Input: part model. Units: mm. Frame: model coordinates. Face numbers are marked on the shaded views. A direction names the side the tool comes from. Give positions to 0.01 mm unless a question says otherwise; leave off trailing zeros. Loops run counter-clockwise (first coordinate to the right, second up) from the corner with the lowest first, then second, coordinate; pieces in that order, holes last. Notation, with made-up numbers: (-34, 20.25) - (6, 20.25) arc R31 cw to (6, 56.25) - close; hole circle Ø3 at (-12, 72.5). An arc over 180 degrees is marked (long way). Answer as a JSON object with one key per item and string values. Group by question number.
(1) Access query for the marked faces 4, 5 and 6. Directions: +Z, -Z, +X, -X, +Y, -Y. A direction counts if a zero-diameter tool reaches every point of the face in a straight line with its end or side. Return the directions, or none.
(2) Section query A-A (y = -28). Return loops of the section in (x, z).
(3) Material intervals for L1, parallel to Z at x = 40.5, y = -23.5; L2, parallel to X at y = -10, z = 9.25; L3, parallel to Z at x = 72, y = 13.5, sorted ascending.
(4) Section query D-D (x = 23.5). Return loops of the section in (y, z).
(5) Section query C-C (y = 44). Return loops of the section in (x, z), plus the area to 3 significant figures.
(6) Pin query (flat end, axial travel): P1, Ø5, axis at x = 5.5, z = 18.5, coming from the -Y side; P2, Ø1.5, axis at y = 22.5, z = 22.5, coming from the -X side; P3, Ø8.5, axis at x = 60.85, y = 12.86, coming from the +Z side. Return the tip coordinate at first contact, or that it passes through.
(7) Section query B-B (z = 16). Return loops of the section in (x, y), plus the area to 3 significant figures.
(8) Mould query, pull axis Z, two halves, no side actions, for the marked faces 1, 2 and 3. Classes: +Z half, -Z half, draft (parallel to the pull), parting line (faces both ways), or undercut.
```python
from build123d import *

# Parameters (mm, degrees)
F1_DEPTH     = 25
F4_DEPTH     = 25
F6_DEPTH     = 20
F7_W         = 51.9104144033
F7_H         = 33.7755738664
F7_W_2       = 52.9833799657
F8_DEPTH     = 25
F9_W         = 5
F9_H         = 24.4488522671
F10_DEPTH    = 20
F11_W        = 120.8302378654
F11_H        = 15
F12_DEPTH    = 30
F14_DEPTH    = 6
F15_R        = 7.2754238601
F15_R_2      = 3.5
F15_R_3      = 6.751082942
F16_DEPTH    = 2
F17_W        = 5
F17_H        = 5
F18_DEPTH    = 58
F19_DEPTH    = 2
F20_T1_DEPTH = 5
F20_T3_DEPTH = 5
F20_T5_DEPTH = 50
F20_T7_DEPTH = 30
F20_T9_DEPTH = 30


# Not quite as in the source:
# - a fillet or chamfer that OpenCascade refuses, or shapes differently, is made with other operations: its cross-section is extruded or revolved along the edge and cut away or added
# - a feature names something its author has since deleted; it is built from what else it names


with BuildPart() as f1:
    # F0 (on Top) → F1 (new body)
    with BuildSketch(Plane.XY):
        Polygon((-25, 55.486739397), (-90.4999962505, 55.486739397), (-90.4999962505, -36.513260603), (90.5000037495, -36.513260603), (90.5000037495, 55.486739397), (25, 55.486739397), align=None)
    extrude(amount=F1_DEPTH)

    # F3 (on face) → F4 (cut)
    with BuildSketch(Plane.XY.offset(25)):
        Polygon((10, -17.952421695), (0, -17.952421695), (-10, -17.952421695), (-10, -30.3189372783), (0, -30.3189372783), (10, -30.3189372783), align=None)
        Polygon((10, -36.513260603), (10, -30.3189372783), (0, -30.3189372783), (-10, -30.3189372783), (-10, -36.513260603), align=None)
    extrude(amount=-F4_DEPTH, mode=Mode.SUBTRACT)

    # F5 (on face) → F6 (cut)
    with BuildSketch(Plane.XY.offset(25)):
        Polygon((83.3136215806, -2.7376867365), (83.3136215806, 55.486739397), (-90.4999962505, 55.486739397), (-90.4999962505, -36.513260603), (-37.5166162848, -36.513260603), (-37.5166162848, -2.7376867365), align=None)
    extrude(amount=-F6_DEPTH, mode=Mode.SUBTRACT)

    # F7 (on face) → F8 (cut)
    with BuildSketch(Plane.XY.offset(5)):
        with Locations((-64.5447890489, 38.5989524638)):
            Rectangle(F7_W, F7_H)
        with Locations((-64.0083062677, -19.6254736697)):
            Rectangle(F7_W_2, F7_H)
    extrude(amount=-F8_DEPTH, mode=Mode.SUBTRACT)

    # F9 (on face) → F10 (join)
    with BuildSketch(Plane.XY.offset(5)):
        with Locations((-87.9999962505, 9.486739397)):
            Rectangle(F9_W, F9_H)
    extrude(amount=F10_DEPTH)

    # F11 (on face) → F12 (cut)
    with BuildSketch(Plane(origin=(0, -2.7376867365, 0), x_dir=(-1, 0, 0), z_dir=(0, 1, 0))):
        with Locations((-22.8985026479, 12.5)):
            Rectangle(F11_W, F11_H)
    extrude(amount=-F12_DEPTH, mode=Mode.SUBTRACT)

    # F13 (on face) → F14 (cut)
    with BuildSketch(Plane.XY.offset(5)):
        with BuildLine():
            ThreePointArc((64.3544293493, 12.8630390391), (60.8544293493, 16.3630390391), (57.3544293493, 12.8630390391))
            Line((57.3544293493, 12.8630390391), (60.8544293493, 12.8630390391))
            Line((60.8544293493, 12.8630390391), (64.3544293493, 12.8630390391))
        make_face()
        with BuildLine():
            Line((60.8544293493, 12.8630390391), (57.3544293493, 12.8630390391))
            ThreePointArc((57.3544293493, 12.8630390391), (60.8544293493, 9.3630390391), (64.3544293493, 12.8630390391))
            Line((64.3544293493, 12.8630390391), (60.8544293493, 12.8630390391))
        make_face()
        with BuildLine():
            ThreePointArc((-23.8955706507, 12.8630390391), (-27.3955706507, 16.3630390391), (-30.8955706507, 12.8630390391))
            Line((-30.8955706507, 12.8630390391), (-27.3955706507, 12.8630390391))
            Line((-27.3955706507, 12.8630390391), (-23.8955706507, 12.8630390391))
        make_face()
        with BuildLine():
            Line((-27.3955706507, 12.8630390391), (-30.8955706507, 12.8630390391))
            ThreePointArc((-30.8955706507, 12.8630390391), (-27.3955706507, 9.3630390391), (-23.8955706507, 12.8630390391))
            Line((-23.8955706507, 12.8630390391), (-27.3955706507, 12.8630390391))
        make_face()
    extrude(amount=-F14_DEPTH, mode=Mode.SUBTRACT)

    # F15 (on face) → F16 (cut)
    with BuildSketch(Plane.XY.offset(5)):
        with Locations((60.8544293493, 12.8630390391)):
            Circle(F15_R)
        with Locations((60.8544293493, 12.8630390391)):
            Circle(F15_R_2, mode=Mode.SUBTRACT)
        with Locations((-27.3955706507, 12.8630390391)):
            Circle(F15_R_3)
        with Locations((-27.3955706507, 12.8630390391)):
            Circle(F15_R_2, mode=Mode.SUBTRACT)
    extrude(amount=-F16_DEPTH, mode=Mode.SUBTRACT)

    # F17 (on face) → F18 (join)
    with BuildSketch(Plane(origin=(0, -2.7376867365, 0), x_dir=(-1, 0, 0), z_dir=(0, 1, 0))):
        with Locations((-80.8136215806, 22.5)):
            Rectangle(F17_W, F17_H)
    extrude(amount=F18_DEPTH)

    # F19 (cut): a face of the model
    f19_faces = [f1.faces().sort_by_distance(p)[0] for p in [
        (83.3136215806, 11.4118039273, 12.5084721811),
    ]]
    extrude(f19_faces, amount=-F19_DEPTH, mode=Mode.SUBTRACT)

    # F20: fillet of radius 5 on 17 edges, made by hand

    # F20_s2 → F20_t1 (join)
    with BuildSketch(Plane.XY.offset(20)):
        with BuildLine():
            ThreePointArc((-10, -22.952421695), (-8.5355339059, -19.4168877891), (-5, -17.952421695))
            Line((-5, -17.952421695), (-10, -17.952421695))
            Line((-10, -17.952421695), (-10, -22.952421695))
        make_face()
        with BuildLine():
            ThreePointArc((5, -17.952421695), (8.5355339059, -19.4168877891), (10, -22.952421695))
            Line((10, -22.952421695), (10, -17.952421695))
            Line((10, -17.952421695), (5, -17.952421695))
        make_face()
        with BuildLine():
            ThreePointArc((78.3136215806, 2.2623132635), (76.8491554865, -1.2732206424), (73.3136215806, -2.7376867365))
            Line((73.3136215806, -2.7376867365), (78.3136215806, -2.7376867365))
            Line((78.3136215806, -2.7376867365), (78.3136215806, 2.2623132635))
        make_face()
    extrude(amount=F20_T1_DEPTH)

    # F20_s4 → F20_t3 (join)
    with BuildSketch(Plane.XY):
        with BuildLine():
            ThreePointArc((-10, -22.952421695), (-8.5355339059, -19.4168877891), (-5, -17.952421695))
            Line((-5, -17.952421695), (-10, -17.952421695))
            Line((-10, -17.952421695), (-10, -22.952421695))
        make_face()
        with BuildLine():
            ThreePointArc((10, -22.952421695), (8.5355339059, -19.4168877891), (5, -17.952421695))
            Line((5, -17.952421695), (10, -17.952421695))
            Line((10, -17.952421695), (10, -22.952421695))
        make_face()
        with BuildLine():
            ThreePointArc((-42.5166162848, -2.7376867365), (-38.9810823789, -4.2021528306), (-37.5166162848, -7.7376867365))
            Line((-37.5166162848, -7.7376867365), (-37.5166162848, -2.7376867365))
            Line((-37.5166162848, -2.7376867365), (-42.5166162848, -2.7376867365))
        make_face()
        with BuildLine():
            ThreePointArc((-38.5895818472, 26.7111655306), (-40.0540479413, 23.1756316247), (-43.5895818472, 21.7111655306))
            Line((-43.5895818472, 21.7111655306), (-38.5895818472, 21.7111655306))
            Line((-38.5895818472, 21.7111655306), (-38.5895818472, 26.7111655306))
        make_face()
    extrude(amount=F20_T3_DEPTH)

    # F20_s6 → F20_t5 (cut)
    with BuildSketch(Plane.XY.offset(-12.5)):
        with BuildLine():
            ThreePointArc((-10, -31.513260603), (-11.4644660941, -35.0487945089), (-15, -36.513260603))
            Line((-15, -36.513260603), (-10, -36.513260603))
            Line((-10, -36.513260603), (-10, -31.513260603))
        make_face()
        with BuildLine():
            ThreePointArc((15, -36.513260603), (11.4644660941, -35.0487945089), (10, -31.513260603))
            Line((10, -31.513260603), (10, -36.513260603))
            Line((10, -36.513260603), (15, -36.513260603))
        make_face()
        with BuildLine():
            ThreePointArc((-32.5166162848, -36.513260603), (-36.0521501908, -35.0487945089), (-37.5166162848, -31.513260603))
            Line((-37.5166162848, -31.513260603), (-37.5166162848, -36.513260603))
            Line((-37.5166162848, -36.513260603), (-32.5166162848, -36.513260603))
        make_face()
        with BuildLine():
            ThreePointArc((90.5000037495, 50.486739397), (89.0355376554, 54.022273303), (85.5000037495, 55.486739397))
            Line((85.5000037495, 55.486739397), (90.5000037495, 55.486739397))
            Line((90.5000037495, 55.486739397), (90.5000037495, 50.486739397))
        make_face()
        with BuildLine():
            ThreePointArc((90.5000037495, -31.513260603), (89.0355376554, -35.0487945089), (85.5000037495, -36.513260603))
            Line((85.5000037495, -36.513260603), (90.5000037495, -36.513260603))
            Line((90.5000037495, -36.513260603), (90.5000037495, -31.513260603))
        make_face()
        with BuildLine():
            ThreePointArc((-90.4999962505, 16.7111655306), (-89.0355301565, 20.2466994365), (-85.4999962505, 21.7111655306))
            Line((-85.4999962505, 21.7111655306), (-90.4999962505, 21.7111655306))
            Line((-90.4999962505, 21.7111655306), (-90.4999962505, 16.7111655306))
        make_face()
        with BuildLine():
            ThreePointArc((-90.4999962505, 2.2623132635), (-89.0355301565, -1.2732206424), (-85.4999962505, -2.7376867365))
            Line((-85.4999962505, -2.7376867365), (-90.4999962505, -2.7376867365))
            Line((-90.4999962505, -2.7376867365), (-90.4999962505, 2.2623132635))
        make_face()
    extrude(amount=F20_T5_DEPTH, mode=Mode.SUBTRACT)

    # F20_s8 → F20_t7 (cut)
    with BuildSketch(Plane.XY.offset(-12.5)):
        with BuildLine():
            ThreePointArc((-33.5895818472, 55.486739397), (-37.1251157531, 54.022273303), (-38.5895818472, 50.486739397))
            Line((-38.5895818472, 50.486739397), (-38.5895818472, 55.486739397))
            Line((-38.5895818472, 55.486739397), (-33.5895818472, 55.486739397))
        make_face()
    extrude(amount=F20_T7_DEPTH, mode=Mode.SUBTRACT)

    # F20_s10 → F20_t9 (cut)
    with BuildSketch(Plane.XY.offset(7.5)):
        with BuildLine():
            ThreePointArc((83.3136215806, 55.2623132635), (79.7780876747, 53.7978471694), (78.3136215806, 50.2623132635))
            Line((78.3136215806, 50.2623132635), (78.3136215806, 55.2623132635))
            Line((78.3136215806, 55.2623132635), (83.3136215806, 55.2623132635))
        make_face()
        with BuildLine():
            ThreePointArc((-37.5166162848, -7.7376867365), (-36.0521501908, -4.2021528306), (-32.5166162848, -2.7376867365))
            Line((-32.5166162848, -2.7376867365), (-37.5166162848, -2.7376867365))
            Line((-37.5166162848, -2.7376867365), (-37.5166162848, -7.7376867365))
        make_face()
    extrude(amount=F20_T9_DEPTH, mode=Mode.SUBTRACT)


solid = f1.part
```
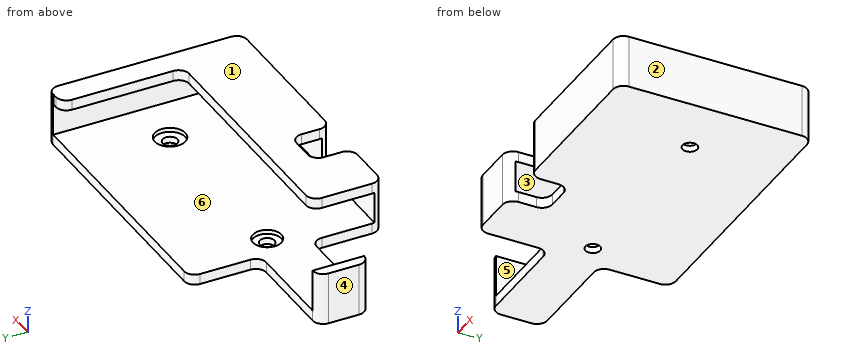
Recorded:
{
 "1": {"face 4": "+Z, -Z, -X, +Y, -Y", "face 5": "+Z, +Y, -Y", "face 6": "+Y"},
 "2": {"outline": "(-37.52, 0) - (-10, 0) - (-10, 5) - (-37.52, 5) - close; (-37.52, 20) - (-10, 20) - (-10, 25) - (-37.52, 25) - close; (10, 0) - (90.5, 0) - (90.5, 25) - (10, 25) - (10, 20) - (85.31, 20) - (85.31, 5) - (10, 5) - close"},
 "3": {"L1": "z = 0 to 5, 20 to 25", "L2": "x = 85.31 to 90.5", "L3": "z = 0 to 5"},
 "4": {"outline": "(-36.51, 0) - (55.49, 0) - (55.49, 5) - (-32.74, 5) - (-32.74, 20) - (-2.74, 20) - (-2.74, 25) - (-36.51, 25) - close"},
 "5": {"outline": "(-38.59, 0) - (90.5, 0) - (90.5, 25) - (78.31, 25) - (78.31, 20) - (85.31, 20) - (85.31, 5) - (-38.59, 5) - close", "area": "784 mm^2"},
 "6": {"P1": "stops at y = -18.62", "P2": "stops at x = 78.31", "P3": "stops at z = 3"},
 "7": {"outline": "(-90.5, 2.26) arc R5 ccw to (-85.5, -2.74) - (-85.5, 21.71) arc R5 ccw to (-90.5, 16.71) - close; (-37.36, -32.74) arc R5 ccw to (-32.52, -36.51) - (-15, -36.51) arc R5 ccw to (-10.15, -32.74) - close; (10.15, -32.74) arc R5 ccw to (15, -36.51) - (85.5, -36.51) arc R5 ccw to (90.5, -31.51) - (90.5, 50.49) arc R5 ccw to (85.5, 55.49) - (85.31, 55.49) - (85.31, -32.74) - close", "area": "950 mm^2"},
 "8": {"face 1": "+Z half", "face 2": "draft", "face 3": "undercut"}
}
